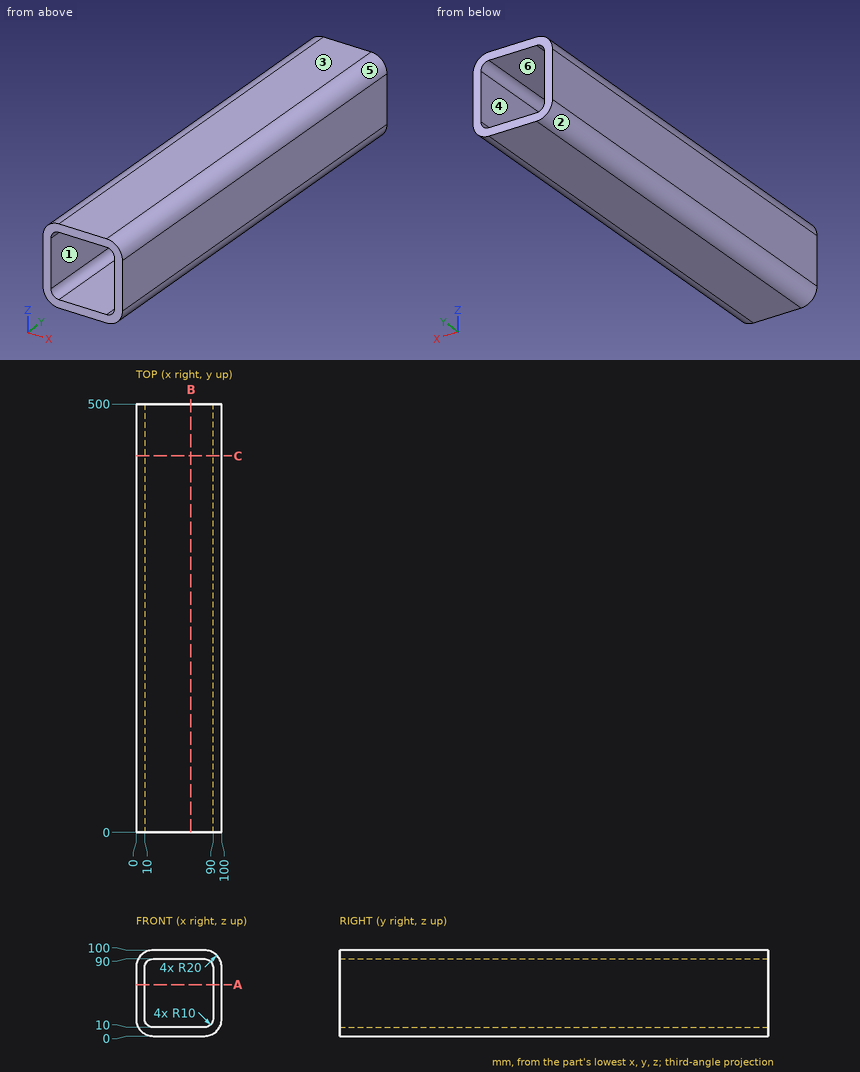
Verification items for this drawing (mm, ordinates from the low corner). A direction names the side the tool comes from. Give positions to 0.01 mm unless a question says otherwise; leave off trailing zeros. Loops run counter-clockwise (first coordinate to the right, second up) from the corner with the lowest first, then second, coordinate; pieces in that order, holes last. Notation, with made-up numbers: M 73.25,49 L 102.25,49 A15 ccw 102.25,70 Z; hole C 30,-27 d3. An arc over 180 degrees is marked long. Answer as a JSON object with one key per item and string values. Group by question number.
Q1. Cross-section at C-C on y = 439.5. Record the cut outline in (x, z), then the cut area to 3 significant figures.
Q2. Go/stop test with flat-tipped pins: P1, Ø3, axis at x = 14.5, y = 73.5, coming from the +Z side; P2, Ø4, axis at x = 85.5, y = 441, coming from the -Z side; P3, Ø18, axis at x = 60, y = 247, coming from the -Z side. Record where each tip stops, or that it passes through.
Q3. Cross-section at A-A on z = 60. Record the cut outline in (x, y), then the cut area to 3 significant figures.
Q4. Release check for a two-part mould opening along X. For the marked faces 1, 2, 3 and 4 record: released by +X, released by -X, zero draft, split by the parting line, or undercut.
Q5. Material ranges on line 1 along X through (y, z) = (161.5, 20.5); line 2 along Z through (x, y) = (82, 448), recorded low to high. Write a range as [from, to].
Q6. Access from +Z, -Z, +X, -X, +Y, -Y to the whole of each face (thin tool, end or side, straight path). Record for the marked faces 5 and 6.
Q7. Cross-section at B-B on x = 64. Record the cut outline in (y, z), then the cut area to 3 significant figures.
Evaluation:
{
 "1": {"outline": "M 0,20 A20 ccw 20,0 L 80,0 A20 ccw 100,20 L 100,80 A20 ccw 80,100 L 20,100 A20 ccw 0,80 Z; hole M 10,20 A10 ccw 20,10 L 80,10 A10 ccw 90,20 L 90,80 A10 ccw 80,90 L 20,90 A10 ccw 10,80 Z", "area": "3,340 mm2"},
 "2": {"P1": "stops at z = 99.6", "P2": "stops at z = 0.31", "P3": "stops at z = 0"},
 "3": {"outline": "M 0,0 L 10,0 L 10,500 L 0,500 Z; M 90,0 L 100,0 L 100,500 L 90,500 Z", "area": "10,000 mm2"},
 "4": {"face 1": "undercut", "face 2": "released by -X", "face 3": "zero draft", "face 4": "undercut"},
 "5": {"line 1": "x = [0, 10], [90, 100]", "line 2": "z = [0.1, 10.2], [89.8, 99.9]"},
 "6": {"face 5": "+Z, +X, +Y, -Y", "face 6": "+Y, -Y"},
 "7": {"outline": "M 0,0 L 500,0 L 500,10 L 0,10 Z; M 0,90 L 500,90 L 500,100 L 0,100 Z", "area": "10,000 mm2"}
}
